Work out the finished part from the listing and answer in its coordinate system (mm). Face numbers are marked on the shaded views. A direction names the side the tool comes from. Give positions to 0.01 mm unless a question says otherwise; leave off trailing zeros. Loops run counter-clockwise (first coordinate to the right, second up) from the corner with the lowest first, then second, coordinate; pieces in that order, holes last. Notation, with made-up numbers: (-7, 76) - (43, 76) arc R14 cw to (43, 95) - close; hole circle Ø9 at (17.5, 60.5). An arc over 180 degrees is marked (long way). One line per question, with ' | ' between items.
from build123d import *

# Parameters (mm, degrees)
SKETCH1_R            = 22.225
SKETCH1_R_2          = 17.4625
SPRING_CHAMBER_DEPTH = 28.575
BALL_CHAMBER_START   = 47.625
SKETCH2_R            = 22.225
SKETCH2_R_2          = 9.525
BALL_CHAMBER_DEPTH   = 47.625
SKETCH5_R            = 3.81
BALL_HOLE_DEPTH      = 58.061737399
SKETCH8_R            = 22.225
SKETCH8_R_2          = 11.90625
CUT_EXTRUDE2_DEPTH   = 41.275


with BuildPart() as part:
    # Sketch1 → spring_chamber (new body)
    with BuildSketch(Plane(origin=(0, 0, 0), x_dir=(1, 0, 0), z_dir=(0, 1, 0))):
        with Locations(Location((0, 0, 0), (0, 0, 270))):
            Circle(SKETCH1_R)
        with Locations(Location((0, 0, 0), (0, 0, 270))):
            Circle(SKETCH1_R_2, mode=Mode.SUBTRACT)
    extrude(amount=SPRING_CHAMBER_DEPTH)

    # Sketch2 → ball_chamber (add)
    with BuildSketch(Plane.XZ.offset(BALL_CHAMBER_START)):
        with Locations(Location((0, 0, 0), (0, 0, 270))):
            Circle(SKETCH2_R)
        with Locations(Location((0, 0, 0), (0, 0, 270))):
            Circle(SKETCH2_R_2, mode=Mode.SUBTRACT)
    extrude(amount=-BALL_CHAMBER_DEPTH)

    # Sketch5 → ball_hole (cut, through all)
    with BuildSketch(Plane(origin=(0, 0, 0), x_dir=(0, 0, -1), z_dir=(1, 0, 0))):
        with Locations(Location((0, -28.575, 0), (0, 0, 180))):
            Circle(SKETCH5_R)
    ball_hole = extrude(amount=BALL_HOLE_DEPTH, mode=Mode.SUBTRACT)

    # Sketch8 → Cut-Extrude2 (cut)
    with BuildSketch(Plane.XZ.offset(47.625)):
        with Locations(Location((0, 0, 0), (0, 0, 270))):
            Circle(SKETCH8_R)
        with Locations(Location((0, 0, 0), (0, 0, 270))):
            Circle(SKETCH8_R_2, mode=Mode.SUBTRACT)
    extrude(amount=-CUT_EXTRUDE2_DEPTH, mode=Mode.SUBTRACT)

    # Mirror1: ball_hole across plane
    add(ball_hole.mirror(Plane(origin=(0, 0, 0), x_dir=(0, 0, 1), z_dir=(1, 0, 0))), mode=Mode.SUBTRACT)


solid = part.part
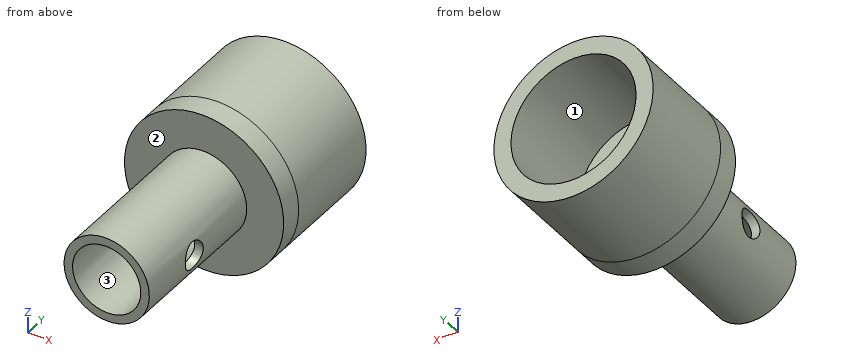
1. Find section C-C on y = -1.5. Write down the section's boundary in (x, z) (3 decimals).
Evaluation:
outline: circle Ø44.45 at (0, 0); hole circle Ø19.05 at (0, 0)
2. Consider L1, parallel to Y at x = -10, z = 0 (3 decimals); L2, parallel to X at y = 18, z = 0 (1 decimal); L3, parallel to Y at x = 14.5, z = 0.5. Determine where each line is inside the solid, lowest interval first.
Evaluation:
L1: -47.625 to -32.385, -24.765 to 0 | L2: -22.2 to -17.5, 17.5 to 22.2 | L3: -6.35 to 0
3. Find section D-D on z = 8. Write down the section's boundary in (x, y) (3 decimals).
Evaluation:
outline: (-20.735, -6.35) - (-8.818, -6.35) - (-8.818, -47.625) - (-5.17, -47.625) - (-5.17, 0) - (-15.522, 0) - (-15.522, 28.575) - (-20.735, 28.575) - close; (5.17, -47.625) - (8.818, -47.625) - (8.818, -6.35) - (20.735, -6.35) - (20.735, 28.575) - (15.522, 28.575) - (15.522, 0) - (5.17, 0) - close
4. Flat-ended cylindrical pins translate along their axes: pin 1 (21 mm diameter, centred on x = 0, z = 0, fed in from +Y); pin 2 (3 mm diameter, centred on y = 6.5, z = 15, fed in from -X); pin 3 (1.5 mm diameter, centred on y = -18.5, z = -3, fed in from -X). Find the tip coordinate at first contact, or state that the pin passes through.
Evaluation:
pin 1: y = 0 | pin 2: x = -17.66 | pin 3: x = -11.69
5. Which of the six approach directions +Z, -Z, +X, -X, +Y, -Y give full straight-line access (tool end or side, diameter ignored) to the marked faces 1, 2 and 3?
Evaluation:
face 1: +Y | face 2: -Y | face 3: +Y, -Y
6. Find section B-B on z = 0. State how many separate pieces and enclosed holes the cut face has, then the cut area to 3 significant figures.
Evaluation:
separate pieces: 4 | enclosed holes: 0 | area: 594 mm2
